Model file for the job. Use its own axes, mm. Round coordinates to 2 decimals unless told otherwise and drop trailing zeros. Write each loop counter-clockwise with the first axis right and the second up, starting at its lowest first coordinate (ties: lowest second). Pieces come first, ordered by that corner, then holes. Notation, with made-up numbers: (64, -19) - (101, -19) arc R9 ccw to (101, -7) - close; hole circle Ø1 at (-33.5, 83.5). An arc over 180 degrees is marked (long way). One line per item, written item: value.
from build123d import *

# Parameters (mm, degrees)
BOSS_EXTRUDE1_DEPTH                               = 6.35
FILLET1_R                                         = 25.4
CSK_FOR_6_FLAT_HEAD_MACHINE_SCREW_100_D           = 4.3053
CSK_FOR_6_FLAT_HEAD_MACHINE_SCREW_100_CSINK_D     = 7.0866
CSK_FOR_6_FLAT_HEAD_MACHINE_SCREW_100_CSINK_ANGLE = 100
CSK_FOR_8_FLAT_HEAD_MACHINE_SCREW_100_D           = 4.9149
CSK_FOR_8_FLAT_HEAD_MACHINE_SCREW_100_CSINK_D     = 8.4328
CSK_FOR_8_FLAT_HEAD_MACHINE_SCREW_100_CSINK_ANGLE = 100
FILLET2_R                                         = 6.35


with BuildPart() as part:
    # Sketch1 → Boss-Extrude1 (new body)
    with BuildSketch(Plane.ZY.offset(-5.035827965)):
        Polygon((-147.77562455, 230.070458845), (-162.269800873, 312.271017517), (-159.04513305, 330.559017517), (-120.626834873, 330.559017517), (-120.626834873, 295.511176933), (-110.25444916, 236.686454414), align=None)
    extrude(amount=BOSS_EXTRUDE1_DEPTH)

    # Fillet1
    fillet1_edges = [part.edges().sort_by_distance(p)[0] for p in [
        (1.860827965, 312.271017517, -162.269800873),
        (1.860827965, 295.511176933, -120.626834873),
    ]]
    fillet(fillet1_edges, radius=FILLET1_R)

    # CSK for #6 Flat Head Machine Screw (100)1 (through all)
    with Locations(Plane.ZY.offset(1.314172035)):
        with Locations((-124.504125043, 273.139415456), (-144.485224025, 269.724179148), (-140.075144867, 244.324179148), (-120.227402214, 247.716621746)):
            CounterSinkHole(CSK_FOR_6_FLAT_HEAD_MACHINE_SCREW_100_D / 2, CSK_FOR_6_FLAT_HEAD_MACHINE_SCREW_100_CSINK_D / 2, counter_sink_angle=CSK_FOR_6_FLAT_HEAD_MACHINE_SCREW_100_CSINK_ANGLE)

    # CSK for #8 Flat Head Machine Screw (100)1 (through all)
    with Locations(Plane.ZY.offset(1.314172035)):
        with Locations((-149.328834873, 320.907017517), (-130.278834873, 308.207017517)):
            CounterSinkHole(CSK_FOR_8_FLAT_HEAD_MACHINE_SCREW_100_D / 2, CSK_FOR_8_FLAT_HEAD_MACHINE_SCREW_100_CSINK_D / 2, counter_sink_angle=CSK_FOR_8_FLAT_HEAD_MACHINE_SCREW_100_CSINK_ANGLE)

    # Fillet2
    fillet2_edges = [part.edges().sort_by_distance(p)[0] for p in [
        (1.860827965, 230.070458845, -147.77562455),
        (1.860827965, 330.559017517, -159.04513305),
        (1.860827965, 330.559017517, -120.626834873),
        (1.860827965, 236.686454414, -110.25444916),
    ]]
    fillet(fillet2_edges, radius=FILLET2_R)


solid = part.part
1. Wall check: probe 1 along Z at (x, y) = (2.75, 323); probe 2 along Z at (x, y) = (3.25, 270); probe 3 along Y at (x, z) = (2, -145). Give the ranges that are in metal, low to high. Write a range as [from, to].
Report:
probe 1: [-160.38, -150.62], [-148.04, -120.63]
probe 2: [-154.82, -146.62], [-142.35, -116.13]
probe 3: [231.54, 267.63], [271.81, 330.56]
2. Band-saw the part on A-A on x = 1.25. Write the cut outline in (y, z), plus the area to 3 significant figures.
Report:
outline: (231.17, -141.52) arc R6.35 ccw to (236.32, -148.88) - (307.86, -161.49) arc R25.4 ccw to (316.68, -161.49) - (325.31, -159.97) arc R6.35 ccw to (330.56, -153.72) - (330.56, -126.98) arc R6.35 ccw to (324.21, -120.63) - (297.73, -120.63) arc R25.4 cw to (293.32, -120.24) - (242.94, -111.36) arc R6.35 ccw to (235.58, -116.51) - close; hole circle Ø4.31 at (244.32, -140.08); hole circle Ø4.31 at (247.72, -120.23); hole circle Ø4.31 at (269.72, -144.49); hole circle Ø4.31 at (273.14, -124.5); hole circle Ø4.91 at (308.21, -130.28); hole circle Ø4.91 at (320.91, -149.33)
area: 3,680 mm²
3. Band-saw the part on B-B on y = 256.5. Write the cut outline in (x, z), plus the area to 3 significant figures.
Report:
outline: (-1.31, -152.44) - (5.04, -152.44) - (5.04, -113.75) - (-1.31, -113.75) - close
area: 246 mm²
4. Band-saw the part on C-C on z = -156.5. Write the cut outline in (x, y).
Report:
outline: (-1.31, 279.55) - (5.04, 279.55) - (5.04, 329.92) - (-1.31, 329.92) - close
5. Drop flat-ended pins along their axis: pin 1 (5 mm diameter, centred on y = 247.72, z = -120.23, fed in from +X); pin 2 (3 mm diameter, centred on x = 0, y = 276.5, fed in from +Z); pin 3 (8 mm diameter, centred on y = 308.21, z = -130.28, fed in from -X). Give the stop position or say it passes through.
Report:
pin 1: x = 5.04
pin 2: z = -117.01
pin 3: x = -1.14
6. Mould opens along Y. For faces 1 (the face through (2.48, 249.85, -119.95)), 2 (the face through (2.481, 271.859, -144.205)), 3 (the face through (1.816, 232.265, -146.324)), 4 (the face through (1.91, 268.48, -115.86)) say: released by +Y, released by -Y, zero draft, split by the parting line, or undercut.
Report:
face 1: undercut
face 2: undercut
face 3: released by -Y
face 4: released by +Y
